Input: part model. Units: mm. Frame: model coordinates. A direction names the side the tool comes from. Round coordinates to 2 decimals unless told otherwise and drop trailing zeros. Order: outer loops, then holes, each group sorted by start corner. A loop starts at its lowest first (then second) coordinate and runs counter-clockwise, first axis right, second up. Notation, with made-up numbers: (59.5, 67) - (64.5, 67) arc R13 ccw to (64.5, 73) - close; hole circle Ø1 at (67, 15.5). An arc over 180 degrees is marked (long way). One line per item, written item: value. Start each with the question number.
from build123d import *

# Parameters (mm, degrees)
SKETCH1_W           = 20
SKETCH1_H           = 20
BOSS_EXTRUDE1_DEPTH = 5
CUT_EXTRUDE1_DEPTH  = 3
SKETCH4_R           = 2.5
CUT_EXTRUDE2_DEPTH  = 3


with BuildPart() as part:
    # Sketch1 → Boss-Extrude1 (new body)
    with BuildSketch(Plane(origin=(0, 0, 0), x_dir=(1, 0, 0), z_dir=(0, 1, 0))):
        Rectangle(SKETCH1_W, SKETCH1_H)
    extrude(amount=BOSS_EXTRUDE1_DEPTH)

    # Sketch3 → Cut-Extrude1 (cut)
    with BuildSketch(Plane(origin=(0, 5, 0), x_dir=(1, 0, 0), z_dir=(0, 1, 0))):
        Polygon((3.92598183, 0), (1.962990915, 3.4), (-1.962990915, 3.4), (-3.92598183, 0), (-1.962990915, -3.4), (1.962990915, -3.4), align=None)
    extrude(amount=-CUT_EXTRUDE1_DEPTH, mode=Mode.SUBTRACT)

    # Sketch4 → Cut-Extrude2 (cut, through all)
    with BuildSketch(Plane(origin=(0, 2, 0), x_dir=(1, 0, 0), z_dir=(0, 1, 0))):
        Circle(SKETCH4_R)
    extrude(amount=-CUT_EXTRUDE2_DEPTH, mode=Mode.SUBTRACT)


solid = part.part
1. Section D-D (x = -2.25). Return the cut outline in (y, z).
2. Line query: line 1 (Z direction, x = 0, y = 0.95); line 2 (Z direction, x = -1, y = 3.65). Output: solid intervals per line, ascending. Write a range as from..to.
3. Pull-direction query (X, two-part tool) for faces 3 (the face through (10, 2, 0)), 4 (the face through (-2, 0, 2)), 5 (the face through (-0.54, 1.01, 2.44)); classes: released by +X, released by -X, zero draft, split by the parting line, or undercut.
4. Section A-A (x = 0). Return the cut outline in (y, z).
5. Pin query (flat end, axial travel): pin 1 (2 mm diameter, centred on x = 1, z = 1.5, fed in from +Y); pin 2 (4.5 mm diameter, centred on x = 0, z = 0, fed in from +Y). Return the tip coordinate at first contact, or that it passes through.
6. Set-up query: faces 1 (the face through (0, 2, -10)), 2 (the face through (-2.931, 3.521, -1.724)). Return all of +Z, -Z, +X, -X, +Y, -Y with unobstructed straight access to the full face (end or side cutting, diameter ignored); none if empty.
7. Section B-B (y = 3.8). Return the cut outline in (x, z), then the cut area to 3 significant figures.
8. Section C-C (z = -2.75). Return the cut outline in (x, y).
Solved:
1. outline: (0, -10) - (5, -10) - (5, -2.9) - (2, -2.9) - (2, -1.09) - (0, -1.09) - close; (0, 1.09) - (2, 1.09) - (2, 2.9) - (5, 2.9) - (5, 10) - (0, 10) - close
2. line 1: z = -10..-2.5, 2.5..10
2. line 2: z = -10..-3.4, 3.4..10
3. face 3: released by +X
3. face 4: zero draft
3. face 5: undercut
4. outline: (0, -10) - (5, -10) - (5, -3.4) - (2, -3.4) - (2, -2.5) - (0, -2.5) - close; (0, 2.5) - (2, 2.5) - (2, 3.4) - (5, 3.4) - (5, 10) - (0, 10) - close
5. pin 1: stops at y = 2
5. pin 2: passes through
6. face 1: -Z, +X, -X, +Y, -Y
6. face 2: +Y
7. outline: (-10, -10) - (10, -10) - (10, 10) - (-10, 10) - close; hole (-3.93, 0) - (-1.96, -3.4) - (1.96, -3.4) - (3.93, 0) - (1.96, 3.4) - (-1.96, 3.4) - close
7. area: 360 mm²
8. outline: (-10, 0) - (10, 0) - (10, 5) - (2.34, 5) - (2.34, 2) - (-2.34, 2) - (-2.34, 5) - (-10, 5) - close
